The drawing under review shows one solid part. Ordinate dimensions are in mm from its lowest x, y, z. A direction names the side the tool comes from. Give positions to 0.01 mm unless a question says otherwise; leave off trailing zeros. Order: outer loops, then holes, each group sorted by start corner. A loop starts at its lowest first (then second) coordinate and runs counter-clockwise, first axis right, second up. Notation, with made-up numbers: (38.25, 61) -> (79.25, 61) arc R19 ccw to (79.25, 89) -> close; hole circle Ø2 at (28, 47). An arc over 180 degrees is marked (long way). One line per item, written item: value.
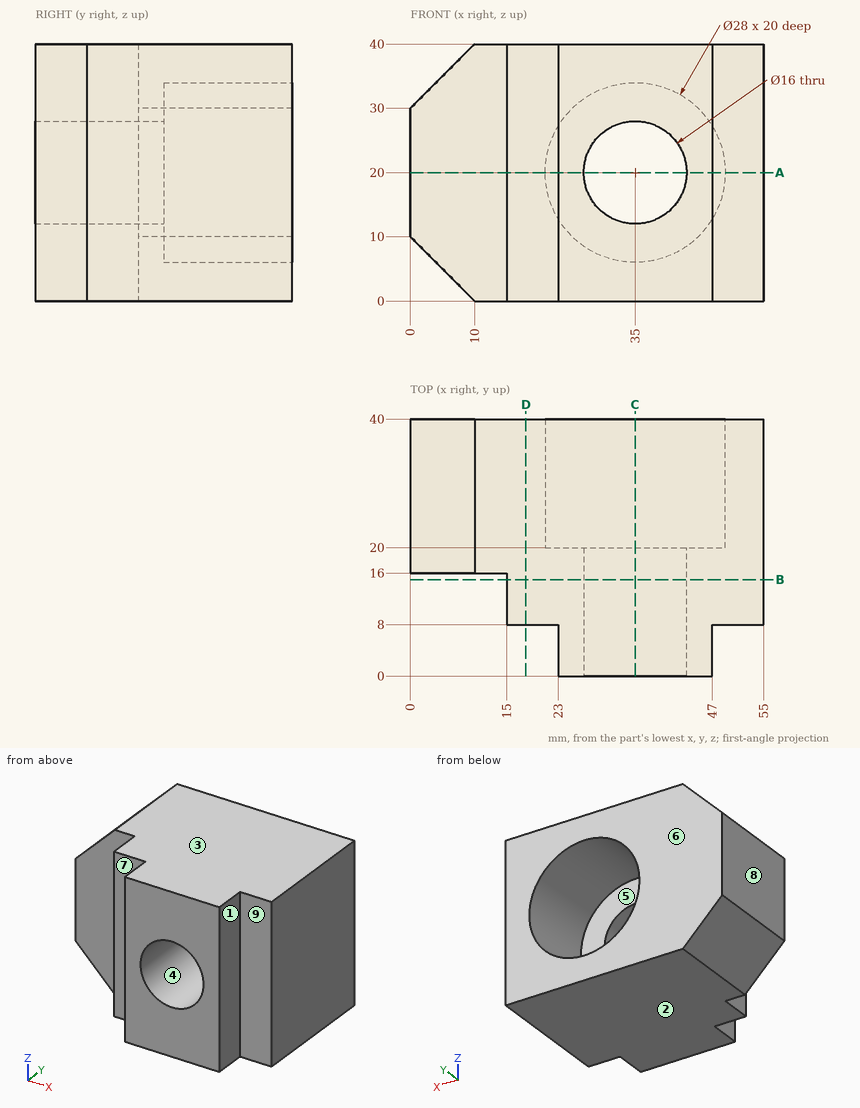
Item 1: Clearance check with flat-ended pins moving along their axes: P1, Ø4, axis at y = 13.5, z = 20, coming from the -X side; P2, Ø4, axis at y = 4.5, z = 15, coming from the +X side; P3, Ø2.5, axis at x = 49, z = 19.5, coming from the -Y side. State where each tip first meets the part, or that it passes through.
Returned:
P1: x = 15
P2: x = 47
P3: y = 8
Item 2: To check wall thickness, follow line 1 along Z through (x, y) = (35, 13); line 2 along Z through (x, y) = (35, 34); line 3 along Y through (x, z) = (52, 12). State the ranges of each line that lie inside material, in increasing order. Write a range as from..to.
Returned:
line 1: 0..12, 28..40
line 2: 0..6, 34..40
line 3: 8..40
Item 3: Add section A-A on z = 20. Give the boundary of the cut face in (x, y).
Returned:
outline: (0, 16) -> (15, 16) -> (15, 8) -> (23, 8) -> (23, 0) -> (27, 0) -> (27, 20) -> (21, 20) -> (21, 40) -> (0, 40) -> close; (43, 0) -> (47, 0) -> (47, 8) -> (55, 8) -> (55, 40) -> (49, 40) -> (49, 20) -> (43, 20) -> close
Item 4: Add section D-D on x = 18. Give the boundary of the cut face in (y, z), plus the area to 3 significant figures.
Returned:
outline: (8, 0) -> (40, 0) -> (40, 40) -> (8, 40) -> close
area: 1,280 mm²
Item 5: Add section C-C on x = 35. Give the boundary of the cut face in (y, z), plus the area to 3 significant figures.
Returned:
outline: (0, 0) -> (40, 0) -> (40, 6) -> (20, 6) -> (20, 12) -> (0, 12) -> close; (0, 28) -> (20, 28) -> (20, 34) -> (40, 34) -> (40, 40) -> (0, 40) -> close
area: 720 mm²
Item 6: Add section B-B on y = 15. Give the boundary of the cut face in (x, z), plus the area to 3 significant figures.
Returned:
outline: (15, 0) -> (55, 0) -> (55, 40) -> (15, 40) -> close; hole circle Ø16 at (35, 20)
area: 1,400 mm²
Item 7: Draft analysis for pull direction Z (two halves, no side actions). For the marked faces 1, 2, 3 and 4, state which applies: pulls with the +Z half, pulls with the -Z half, needs draft (parallel to the pull), parting line crosses it, or undercut.
Returned:
face 1: needs draft
face 2: pulls with the -Z half
face 3: pulls with the +Z half
face 4: undercut
Item 8: Machinability: for the marked faces 5, 6, 7, 8 and 9, which of the approach directions +Z, -Z, +X, -X, +Y, -Y give a long, thin tool a straight path to every point of the face, cutting with its end or side? Answer none if there is none.
Returned:
face 5: +Y
face 6: +Z, -Z, +X, -X, +Y
face 7: +Z, -Z, -X, -Y
face 8: +Z, -Z, -X, +Y, -Y
face 9: +Z, -Z, +X, -Y
